Geometry check sheet. Reference: the model listing, model coordinates, mm. Face numbers are marked on the shaded views. A direction names the side the tool comes from. Coordinates: 2 decimals unless noted, no trailing zeros. Write each loop counter-clockwise with the first axis right and the second up, starting at its lowest first coordinate (ties: lowest second). Pieces come first, ordered by that corner, then holes.
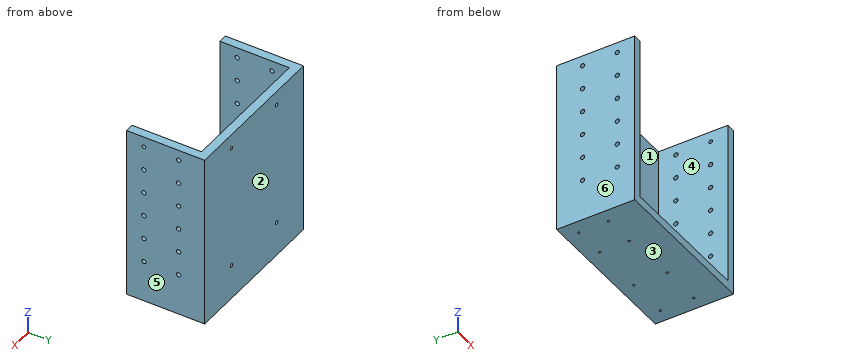
from build123d import *

# Parameters (mm, degrees)
F0_W      = 228.6
F0_H      = 254
F1_DEPTH  = 12.7
F3_DEPTH  = 101.6
F4_R      = 2.667
F4_R_2    = 2.381555
F5_DEPTH  = 25.4
F7_R      = 3.1877
F8_DEPTH  = 25.4
F6_R      = 3.1877
F6_R_2    = 2.750912
F9_DEPTH  = 25.4
F10_R     = 1.5875
F11_DEPTH = 12.701


with BuildPart() as f1:
    # F0 (on Front) → F1 (new body)
    with BuildSketch(Plane.XZ):
        with Locations((5.549081, 26.375307)):
            Rectangle(F0_W, F0_H)
    extrude(amount=F1_DEPTH)

    # F2 (on face) → F3 (join)
    with BuildSketch(Plane.XZ.offset(12.7)):
        Polygon((-96.050919, 153.375307), (-108.750919, 153.375307), (-108.750919, -100.624693), (119.849081, -100.624693), (119.849081, 153.375307), (107.149081, 153.375307), (107.149081, -87.924693), (-96.050919, -87.924693), align=None)
    extrude(amount=F3_DEPTH)

    # F4 (on face) → F5 (cut)
    with BuildSketch(Plane.XZ.offset(12.7)):
        with Locations((-46.647919, 132.445707)):
            Circle(F4_R)
        with Locations((57.746081, 132.445707)):
            Circle(F4_R_2)
        with Locations((57.746081, -49.824693)):
            Circle(F4_R)
        with Locations((-46.647919, -49.824693)):
            Circle(F4_R)
    extrude(amount=-F5_DEPTH, mode=Mode.SUBTRACT)

    # F7 (on face) → F8 (cut)
    with BuildSketch(Plane.YZ.offset(-96.050919)):
        with Locations((-88.9, 102.575307)):
            Circle(F7_R)
        with Locations((-88.9, 138.135307)):
            Circle(F7_R)
        with Locations((-38.1, 138.135307)):
            Circle(F7_R)
        with Locations((-38.1, 102.575307)):
            Circle(F7_R)
        with Locations((-38.1, 67.015307)):
            Circle(F7_R)
        with Locations((-88.9, 67.015307)):
            Circle(F7_R)
        with Locations((-38.1, 31.455307)):
            Circle(F7_R)
        with Locations((-88.9, 31.455307)):
            Circle(F7_R)
        with Locations((-88.9, -39.664693)):
            Circle(F7_R)
        with Locations((-88.9, -4.104693)):
            Circle(F7_R)
        with Locations((-38.1, -4.104693)):
            Circle(F7_R)
        with Locations((-38.1, -39.664693)):
            Circle(F7_R)
    extrude(amount=-F8_DEPTH, mode=Mode.SUBTRACT)

    # F6 (on face) → F9 (cut)
    with BuildSketch(Plane(origin=(107.149081, 0, 0), x_dir=(0, -1, 0), z_dir=(-1, 0, 0))):
        with Locations((38.1, 138.135307)):
            Circle(F6_R)
        with Locations((88.9, 138.135307)):
            Circle(F6_R_2)
        with Locations((38.1, 102.575307)):
            Circle(F6_R)
        with Locations((88.9, 102.575307)):
            Circle(F6_R)
        with Locations((38.1, 67.015307)):
            Circle(F6_R)
        with Locations((88.9, 67.015307)):
            Circle(F6_R)
        with Locations((38.1, 31.455307)):
            Circle(F6_R)
        with Locations((88.9, 31.455307)):
            Circle(F6_R)
        with Locations((38.1, -4.104693)):
            Circle(F6_R)
        with Locations((88.9, -4.104693)):
            Circle(F6_R)
        with Locations((38.1, -39.664693)):
            Circle(F6_R)
        with Locations((88.9, -39.664693)):
            Circle(F6_R)
    extrude(amount=-F9_DEPTH, mode=Mode.SUBTRACT)

    # F10 (on face) → F11 (cut, through all)
    with BuildSketch(Plane.XY.offset(-87.924693)):
        with Locations((38.911981, -19.8501)):
            Circle(F10_R)
        with Locations((99.948181, -19.8501)):
            Circle(F10_R)
        with Locations((99.948181, -68.6943)):
            Circle(F10_R)
        with Locations((38.911981, -68.6943)):
            Circle(F10_R)
        with Locations((-40.767819, -20.0406)):
            Circle(F10_R)
        with Locations((-40.767819, -63.2714)):
            Circle(F10_R)
        with Locations((-88.596019, -63.2714)):
            Circle(F10_R)
        with Locations((-88.596019, -20.0406)):
            Circle(F10_R)
    extrude(amount=-F11_DEPTH, mode=Mode.SUBTRACT)


solid = f1.part
1. Gauge pin test, flat ends, axial feed: pin 1 Ø5.5 at (y, z) = (-88.9, -4.1) entering from +X; pin 2 Ø1.5 at (x, y) = (16.5, -78.5) entering from +Z; pin 3 Ø2 at (x, z) = (-31, 35.5) entering from -Y. Record the tip position at first contact, or that the pin passes through.
Computed values:
pin 1: passes through
pin 2: stops at z = -87.92
pin 3: stops at y = -12.7
2. Sectioned sample at B-B, the plane x = -59. Record the boundary of the cut face in (y, z), and give its area (3 significant figures).
Computed values:
outline: (-114.3, -100.62) - (0, -100.62) - (0, 153.38) - (-12.7, 153.38) - (-12.7, -87.92) - (-114.3, -87.92) - close
area: 4,520 mm2
3. Thickness scan on line 1 along X through (y, z) = (-99, -43); line 2 along Y through (x, z) = (-22, 89); line 3 along Z through (x, y) = (52.5, -53). Record the ranges inside material, lowest first.
Computed values:
line 1: x = -108.75 to -96.05, 107.15 to 119.85
line 2: y = -12.7 to 0
line 3: z = -100.62 to -87.92
4. Access from +Z, -Z, +X, -X, +Y, -Y to the whole of each face (thin tool, end or side, straight path). Record for the marked faces 1 and 2.
Computed values:
face 1: +Z, -Y
face 2: +Z, -Z, +X, -X, +Y
5. Sectioned sample at C-C, the plane z = -66. Record the boundary of the cut face in (x, y), and give its area (3 significant figures).
Computed values:
outline: (-108.75, -114.3) - (-96.05, -114.3) - (-96.05, -12.7) - (107.15, -12.7) - (107.15, -114.3) - (119.85, -114.3) - (119.85, 0) - (-108.75, 0) - close
area: 5,480 mm2
6. Draft check along X on the marked faces 3, 4, 5 and 6. Enter one of: released by +X, released by -X, zero draft, split by the parting line, or undercut.
Computed values:
face 3: zero draft
face 4: undercut
face 5: released by +X
face 6: released by -X
7. Sectioned sample at A-A, the plane y = -31. Record the boundary of the cut face in (x, z), and give its area (3 significant figures).
Computed values:
outline: (-108.75, -100.62) - (119.85, -100.62) - (119.85, 153.38) - (107.15, 153.38) - (107.15, -87.92) - (-96.05, -87.92) - (-96.05, 153.38) - (-108.75, 153.38) - close
area: 9,030 mm2
